For this review, take the finished solid that the model builds, in its own axes (mm). Face numbers are marked on the shaded views. A direction names the side the tool comes from. Give positions to 0.01 mm unless a question says otherwise; leave off trailing zeros. Order: outer loops, then holes, each group sorted by start corner. A loop starts at its lowest first (then second) coordinate and runs counter-clockwise, first axis right, second up. Notation, with made-up numbers: (56.5, -26) - (62.5, -26) arc R7 cw to (62.5, -14) - close; hole circle Ø2 at (19, -22.5). An arc over 180 degrees is marked (long way). Put each result on its own line as item: value. Start each with the question number.
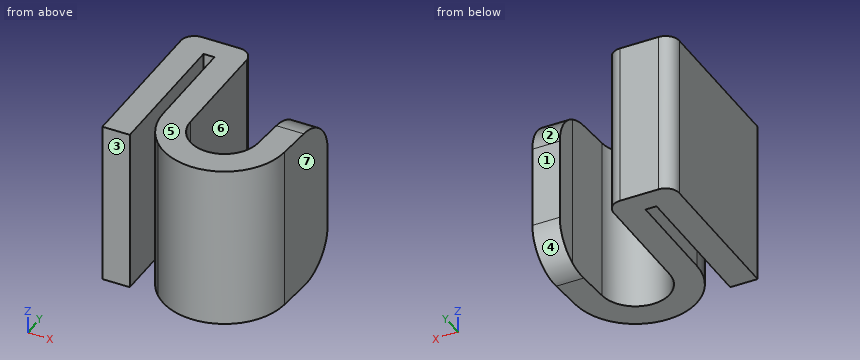
```python
from build123d import *

# Parameters (mm, degrees)
F1_DEPTH = 12
F2_R     = 3
F3_R     = 1


with BuildPart() as f1:
    # F0 (on Top) → F1 (new body)
    with BuildSketch(Plane.XY):
        with BuildLine():
            Line((0, 12), (0, 0))
            Line((0, 0), (2, 0))
            Line((2, 0), (2, 10.3529319381))
            Line((2, 10.3529319381), (2.8, 10.3529319381))
            Line((2.8, 10.3529319381), (2.8, 3.1129138079))
            ThreePointArc((2.8, 3.1129138079), (3.3313730334, 5.2342341514), (4.8, 6.8545711946))
            Line((4.8, 6.8545711946), (4.8, 12))
            Line((4.8, 12), (0, 12))
        make_face()
        with BuildLine():
            Line((4.8, 3.1129138079), (4.8, 6.8545711946))
            ThreePointArc((4.8, 6.8545711946), (3.3313730334, 5.2342341514), (2.8, 3.1129138079))
            ThreePointArc((2.8, 3.1129138079), (3.1242899865, 1.4355808405), (4.0504203926, 0))
            Line((4.0504203926, 0), (4.8, 0))
            Line((4.8, 0), (4.8, 3.1129138079))
        make_face()
        with BuildLine():
            ThreePointArc((9.7952816589, 2.9593903809), (7.2232020421, 0.6140936715), (4.8, 3.1129138079))
            Line((4.8, 3.1129138079), (4.8, 0))
            Line((4.8, 0), (4.0504203926, 0))
            ThreePointArc((4.0504203926, 0), (8.8497267048, -1.1118166144), (11.7916968676, 2.83967536))
            ThreePointArc((11.7916968676, 2.83967536), (11.7979237379, 2.9762315199), (11.8, 3.1129138079))
            ThreePointArc((11.8, 3.1129138079), (11.3319192193, 5.1113200252), (10.0250544847, 6.6939860014))
            Line((10.0250544847, 6.6939860014), (9.7952816589, 2.9593903809))
        make_face()
        with BuildLine():
            Line((10.1232885867, 8.290626709), (10.0250544847, 6.6939860014))
            ThreePointArc((10.0250544847, 6.6939860014), (11.3319192193, 5.1113200252), (11.8, 3.1129138079))
            ThreePointArc((11.8, 3.1129138079), (11.7979237379, 2.9762315199), (11.7916968676, 2.83967536))
            Line((11.7916968676, 2.83967536), (12.1232885867, 8.290626709))
            Line((12.1232885867, 8.290626709), (10.1232885867, 8.290626709))
        make_face()
    extrude(amount=F1_DEPTH)

    # F2
    f2_edges = [f1.edges().sort_by_distance(p)[0] for p in [
        (11.123289, 8.290627, 12),
        (11.123289, 8.290627, 0),
    ]]
    fillet(f2_edges, radius=F2_R)

    # F3
    f3_edges = [f1.edges().sort_by_distance(p)[0] for p in [
        (0, 12, 6),
        (4.8, 12, 6),
    ]]
    fillet(f3_edges, radius=F3_R)


solid = f1.part
```
1. Add section D-D, the plane x = 7.3. Give the boundary of the cut face in (y, z), then the cut area to 3 significant figures.
2. Add section B-B, the plane z = 8.5. Give the boundary of the cut face in (x, y).
3. Tool access review of the marked faces 1, 2, 3 and 4: name each direction out of +Z, -Z, +X, -X, +Y, -Y from which nothing blocks a thin tool from reaching the whole face with its end or side.
4. Add section C-C, the plane y = 1. Give the boundary of the cut face in (x, z), then the cut area to 3 significant figures.
5. Add section A-A, the plane y = 8.5. Give the boundary of the cut face in (x, z), then the cut area to 3 significant figures.
6. Clearance check with flat-ended pins moving along their axes: pin 1 (2 mm diameter, centred on x = 5.5, z = 9, fed in from +Y); pin 2 (2 mm diameter, centred on x = 9.5, z = 3.5, fed in from -Y); pin 3 (0.6 mm diameter, centred on x = 1, z = 5.5, fed in from -Y). State where each tip first meets the part, or that it passes through.
7. Wall thickness on line 1 (X direction, y = 7.5, z = 7); line 2 (X direction, y = 5.5, z = 9.5); line 3 (Y direction, x = 2.25, z = 11.5): over which ranges is each line inside the solid? List them lowest first. Write a range as from..to.
8. The part is to be moulded in two halves that separate along X. For the marked faces 5, 6 and 7, say which applies: released by +X, released by -X, zero draft, split by the parting line, or undercut.
Found:
1. outline: (-1.39, 0) - (0.61, 0) - (0.61, 12) - (-1.39, 12) - close
1. area: 24.0 mm^2
2. outline: (0, 0) - (2, 0) - (2, 10.35) - (2.8, 10.35) - (2.8, 3.11) arc R4.5 ccw to (11.79, 2.84) - (12.12, 8.29) - (10.12, 8.29) - (9.8, 2.96) arc R2.5 cw to (4.8, 3.11) - (4.8, 11) arc R1 ccw to (3.8, 12) - (1, 12) arc R1 ccw to (0, 11) - close
3. face 1: +Z, -Z, +X, +Y
3. face 2: +Z, +X, +Y
3. face 3: +Z, -Z, -X, -Y
3. face 4: -Z, +X, +Y
4. outline: (0, 0) - (2, 0) - (2, 12) - (0, 12) - close; (3.33, 0) - (5.96, 0) - (5.96, 12) - (3.33, 12) - close; (8.64, 0) - (11.27, 0) - (11.27, 12) - (8.64, 12) - close
4. area: 87.3 mm^2
5. outline: (0, 0) - (2, 0) - (2, 12) - (0, 12) - close; (2.8, 0) - (4.8, 0) - (4.8, 12) - (2.8, 12) - close
5. area: 48.0 mm^2
6. pin 1: stops at y = 11.71
6. pin 2: stops at y = -1.22
6. pin 3: stops at y = 0
7. line 1: x = 0..2, 2.8..4.8, 10.07..12.08
7. line 2: x = 0..2, 2.8..4.8, 9.95..11.95
7. line 3: y = 10.35..12
8. face 5: zero draft
8. face 6: undercut
8. face 7: released by +X
